```python
from build123d import *

# Parameters (mm, degrees)
SKETCH1_W           = 107.6
SKETCH1_H           = 59.3
BOSS_EXTRUDE1_DEPTH = 3
SKETCH2_W           = 95.2
SKETCH2_H           = 2.5
SKETCH2_W_2         = 2.5
SKETCH2_H_2         = 46.9
BOSS_EXTRUDE2_DEPTH = 3
SKETCH3_R           = 1.5
SKETCH3_R_2         = 6
SKETCH3_R_3         = 6.557552613
SKETCH3_W           = 31.6
SKETCH3_H           = 15.3
CUT_EXTRUDE1_DEPTH  = 5


with BuildPart() as part:
    # Sketch1 → Boss-Extrude1 (new body)
    with BuildSketch(Plane.XY):
        with Locations((53.8, 29.65)):
            Rectangle(SKETCH1_W, SKETCH1_H)
    extrude(amount=BOSS_EXTRUDE1_DEPTH)

    # Sketch2 → Boss-Extrude2 (add)
    with BuildSketch(Plane.XY.offset(3)):
        with Locations((53.8, 55.85)):
            Rectangle(SKETCH2_W, SKETCH2_H)
        with Locations((3.45, 29.65)):
            Rectangle(SKETCH2_W_2, SKETCH2_H_2)
        with Locations((53.8, 3.45)):
            Rectangle(SKETCH2_W, SKETCH2_H)
        with Locations((104.15, 29.65)):
            Rectangle(SKETCH2_W_2, SKETCH2_H_2)
    extrude(amount=BOSS_EXTRUDE2_DEPTH)

    # Sketch3 → Cut-Extrude1 (cut)
    with BuildSketch(Plane(origin=(0, 0, 0), x_dir=(-1, 0, 0), z_dir=(0, 0, -1))):
        with Locations((-104.6, 56.3)):
            Circle(SKETCH3_R)
        with Locations((-3, 56.3)):
            Circle(SKETCH3_R)
        with Locations((-3, 3)):
            Circle(SKETCH3_R)
        with Locations((-104.6, 3)):
            Circle(SKETCH3_R)
        with Locations((-85.1, 15)):
            Circle(SKETCH3_R_2)
        with Locations((-40.1, 15)):
            Circle(SKETCH3_R_3)
        with Locations((-59.8, 36.65)):
            Rectangle(SKETCH3_W, SKETCH3_H)
    extrude(amount=-CUT_EXTRUDE1_DEPTH, mode=Mode.SUBTRACT)


solid = part.part
```
Here's how the part is built. I have some questions about the finished solid (model axes, mm). A direction names the side the tool comes from. Coordinates: 2 decimals unless noted, no trailing zeros. Loops run counter-clockwise (first coordinate to the right, second up) from the corner with the lowest first, then second, coordinate; pieces in that order, holes last. Notation, with made-up numbers: (86, 34.5) - (123, 34.5) arc R29 ccw to (123, 70.5) - close; hole circle Ø6 at (67, -39). An arc over 180 degrees is marked (long way). Return JSON: item names as keys, results as strings. Group by question number.
Item 1: If we section it at C-C on y = 38: Write out the boundary of the cut face in (x, z), and give its area (3 significant figures).
Item 2: On a 3-axis mill with a long thin cutter (end or side, diameter ignored), from which of +Z, -Z, +X, -X, +Y, -Y can I reach the whole of each face in a straight line? I mean faces 1 (the face through (3, 6.2, 4)), 2 (the face through (3, 53.1, 4)), 3 (the face through (4.7, 29, 4)), 4 (the face through (3, 30, 6)), 5 (the face through (60, 44.3, 1)). Say none if no direction works.
Item 3: If we section it at D-D on y = 14: Write out the boundary of the cut face in (x, z).
Item 4: If we section it at B-B on x = 40.1: Write out the boundary of the cut face in (y, z).
Item 5: Will these pins go through, and if not, where does the flat tip stop? P1, Ø10, axis at x = 70, y = 18, coming from the +Z side; P2, Ø2.5, axis at y = 30.5, z = 5, coming from the +X side; P3, Ø0.9, axis at x = 63.5, z = 5, coming from the +Y side.
Item 6: We'd pull the mould along X, two halves only. Please class faces 6 (the face through (104, 6.2, 4)), 7 (the face through (102.9, 29, 4)), 8 (the face through (2.2, 29, 4)): +X half, -X half, draft (parallel to the pull), parting line (faces both ways), or undercut.
Item 7: If we section it at A-A on z = 5.05: Write out the boundary of the cut face in (x, y).
Item 8: I need wall thicknesses on line 1 (Y direction, x = 3, z = 1.15); line 2 (Y direction, x = 34, z = 3.7); line 3 (X direction, y = 34, z = 0.75). Which ranges of each line are inside material? Lowest first, please. Write a range as from..to.
Calculated:
{
 "1": {"outline": "(0, 0) - (44, 0) - (44, 3) - (4.7, 3) - (4.7, 6) - (2.2, 6) - (2.2, 3) - (0, 3) - close; (75.6, 0) - (107.6, 0) - (107.6, 3) - (105.4, 3) - (105.4, 6) - (102.9, 6) - (102.9, 3) - (75.6, 3) - close", "area": "243 mm^2"},
 "2": {"face 1": "+Z, +X, -X, -Y", "face 2": "+Z, +X, -X, +Y", "face 3": "+Z, +Y, -Y", "face 4": "+Z, +X, -X, +Y, -Y", "face 5": "+Z, -Z"},
 "3": {"outline": "(0, 0) - (33.62, 0) - (33.62, 3) - (4.7, 3) - (4.7, 6) - (2.2, 6) - (2.2, 3) - (0, 3) - close; (46.58, 0) - (79.18, 0) - (79.18, 3) - (46.58, 3) - close; (91.02, 0) - (107.6, 0) - (107.6, 3) - (105.4, 3) - (105.4, 6) - (102.9, 6) - (102.9, 3) - (91.02, 3) - close"},
 "4": {"outline": "(0, 0) - (8.44, 0) - (8.44, 3) - (4.7, 3) - (4.7, 6) - (2.2, 6) - (2.2, 3) - (0, 3) - close; (21.56, 0) - (59.3, 0) - (59.3, 3) - (57.1, 3) - (57.1, 6) - (54.6, 6) - (54.6, 3) - (21.56, 3) - close"},
 "5": {"P1": "stops at z = 3", "P2": "stops at x = 105.4", "P3": "stops at y = 57.1"},
 "6": {"face 6": "draft", "face 7": "undercut", "face 8": "-X half"},
 "7": {"outline": "(2.2, 6.2) - (4.7, 6.2) - (4.7, 53.1) - (2.2, 53.1) - close; (6.2, 2.2) - (101.4, 2.2) - (101.4, 4.7) - (6.2, 4.7) - close; (6.2, 54.6) - (101.4, 54.6) - (101.4, 57.1) - (6.2, 57.1) - close; (102.9, 6.2) - (105.4, 6.2) - (105.4, 53.1) - (102.9, 53.1) - close"},
 "8": {"line 1": "y = 0..1.5, 4.5..54.8, 57.8..59.3", "line 2": "y = 2.2..4.7, 54.6..57.1", "line 3": "x = 0..44, 75.6..107.6"}
}
